```python
from build123d import *

# Parameters (mm, degrees)
F0_R     = 63.5
F1_DEPTH = 127
F2_R     = 50.8
F3_DEPTH = 114.3
F6_R     = 38.1
F6_R_2   = 31.75
F7_DEPTH = 19.05


with BuildPart() as f1:
    # F0 (on Front) → F1 (new body)
    with BuildSketch(Plane.XZ):
        Circle(F0_R)
    extrude(amount=F1_DEPTH)

    # F2 (on Front) → F3 (cut)
    with BuildSketch(Plane.XZ):
        Circle(F2_R)
    extrude(amount=F3_DEPTH, mode=Mode.SUBTRACT)

    # F6 (on Top) → F7 (join)
    with BuildSketch(Plane.XY):
        with Locations((88.1370286467, -48.5165871287)):
            Circle(F6_R)
        with Locations((88.1370286467, -48.5165871287)):
            Circle(F6_R_2, mode=Mode.SUBTRACT)
    extrude(amount=F7_DEPTH)


solid = f1.part
```
Work out the finished part from the listing and answer in its coordinate system (mm). A direction names the side the tool comes from. Coordinates: 2 decimals unless noted, no trailing zeros. Write each loop counter-clockwise with the first axis right and the second up, starting at its lowest first coordinate (ties: lowest second). Pieces come first, ordered by that corner, then holes.
Q1. Each of these flat-tipped pins is pushed along its axis until it touches: pin 1 Ø0.6 at (x, y) = (50.5, -51.5) entering from -Z; pin 2 Ø1 at (y, z) = (-81.5, -9) entering from -X; pin 3 Ø1.5 at (y, z) = (-46, -24) entering from -X. Where does it stop, or does it pass through?
Q2. A cutting plane is placed at A-A, the plane x = 106. Give the vertices of the cut face in (y, z), then the cut area to 3 significant figures.
Q3. Determine the mould class of faces 1 (the face through (-29, 0, 43)), 2 (the face through (-13.77, -62.61, -61.99)), 3 (the face through (-1, -114.3, 1)) for opening direction Z: released by +Z, released by -Z, zero draft, split by the parting line, or undercut.
Q4. Which of the six approach directions +Z, -Z, +X, -X, +Y, -Y give full straight-line access (tool end or side, diameter ignored) to faces 4 (the face through (120, -51, 19.05)), 5 (the face through (-1, -127, 1)), 6 (the face through (120, -46, 0)), 7 (the face through (50.037, -48.41, 3.35))?
Q5. A cutting plane is placed at B-B, the plane x = 0. Give the vertices of the cut face in (y, z), then the cut area to 3 significant figures.
Q6. A cutting plane is placed at C-C, the plane z = 28.5. Give the vertices of the cut face in (x, y).
Q7. Find the intervals of material crossed by line 1 (Z direction, x = 0, y = -60); line 2 (X direction, y = -70, z = -1.5); line 3 (X direction, y = -67, z = 12.5), in increasing order.
Q8. A cutting plane is placed at D-D, the plane z = 5.5. Give the vertices of the cut face in (x, y), then the cut area to 3 significant figures.
Findings below:
1. pin 1: stops at z = -38.89
1. pin 2: stops at x = -62.93
1. pin 3: stops at x = -59.09
2. outline: (-82.17, 0) - (-74.76, 0) - (-74.76, 19.05) - (-82.17, 19.05) - close; (-22.27, 0) - (-14.86, 0) - (-14.86, 19.05) - (-22.27, 19.05) - close
2. area: 282 mm2
3. face 1: zero draft
3. face 2: split by the parting line
3. face 3: undercut
4. face 4: +Z, +X, +Y, -Y
4. face 5: +Z, -Z, +X, -X, -Y
4. face 6: -Z, +X, +Y, -Y
4. face 7: none
5. outline: (-127, -63.5) - (0, -63.5) - (0, -50.8) - (-114.3, -50.8) - (-114.3, 50.8) - (0, 50.8) - (0, 63.5) - (-127, 63.5) - close
5. area: 4,520 mm2
6. outline: (-56.75, -127) - (56.75, -127) - (56.75, 0) - (42.05, 0) - (42.05, -114.3) - (-42.05, -114.3) - (-42.05, 0) - (-56.75, 0) - close
7. line 1: z = -63.5 to -50.8, 50.8 to 63.5
7. line 2: x = -63.48 to -50.78, 50.78 to 63.48
7. line 3: x = -62.26 to -49.24, 49.24 to 62.32, 113.95 to 121.45
8. outline: (-63.26, -127) - (63.26, -127) - (63.26, -77.38) arc R38.1 ccw (long way) to (63.26, -19.66) - (63.26, 0) - (50.5, 0) - (50.5, -42.59) arc R38.1 ccw to (50.5, -54.45) - (50.5, -114.3) - (-50.5, -114.3) - (-50.5, 0) - (-63.26, 0) - close; hole (63.26, -68.25) arc R31.75 ccw (long way) to (63.26, -28.79) - close
8. area: 5,580 mm2
